Read the model definition and answer for the solid it produces. Units are mm, in the model's axes. A direction names the side the tool comes from. Give positions to 0.01 mm unless a question says otherwise; leave off trailing zeros. Order: outer loops, then holes, each group sorted by start corner. A loop starts at its lowest first (then second) coordinate and runs counter-clockwise, first axis right, second up.
```python
from build123d import *

# Parameters (mm, degrees)
F1_DEPTH      = 4.5
F2_DEPTH      = 4
F3_T          = -2.5
F4_R          = 1.52
F5_DEPTH      = 1.04
F6_R          = 1.52
F7_DEPTH      = 1.04
F8_R          = 1.52
F9_DEPTH      = 1.04
F10_R         = 1.52
F11_DEPTH     = 1.04
F12_R         = 1.52
F13_DEPTH     = 1.04
F14_R         = 1.52
F15_DEPTH     = 1.04
F16_T1_DEPTH  = 25.1433659759
F16_T3_DEPTH  = 25.1433659759
F16_T5_DEPTH  = 25.1433659759
F16_T7_DEPTH  = 25.1433659759
F16_T9_DEPTH  = 25.1433659759
F16_T11_DEPTH = 25.1433659759


# Not quite as in the source:
# - a fillet or chamfer that OpenCascade refuses, or shapes differently, is made with other operations: its cross-section is extruded or revolved along the edge and cut away or added


with BuildPart() as f1:
    # F0 (on Top) → F1 (new body)
    with BuildSketch(Plane.XY):
        Polygon((-8.9919036831, 15.2349256124), (-17.6897844467, -0.1697542118), (-8.6978807636, -15.4046798242), (8.9919036831, -15.2349256124), (17.6897844467, 0.1697542118), (8.6978807636, 15.4046798242), align=None)
    extrude(amount=F1_DEPTH)

    # F0 (on Top) → F2 (join)
    with BuildSketch(Plane.XY):
        Polygon((-19.9990791985, -0.1919146011), (-9.8333366793, -17.4156679387), (10.1657425191, -17.2237533376), (19.9990791985, 0.1919146011), (9.8333366793, 17.4156679387), (-10.1657425191, 17.2237533376), align=None)
        Polygon((-8.6978807636, -15.4046798242), (-17.6897844467, -0.1697542118), (-8.9919036831, 15.2349256124), (8.6978807636, 15.4046798242), (17.6897844467, 0.1697542118), (8.9919036831, -15.2349256124), align=None, mode=Mode.SUBTRACT)
    extrude(amount=F2_DEPTH)

    # F3
    f3_openings = [f1.faces().sort_by_distance(p)[0] for p in [
        (0, 0, 0),
    ]]
    offset(amount=F3_T, openings=f3_openings, kind=Kind.INTERSECTION)

    # F4 (on face) → F5 (cut)
    with BuildSketch(Plane(origin=(15.0824108588, -8.5159193683, 0), x_dir=(0.491666834, 0.8707833969, 0), z_dir=(0.8707833969, -0.491666834, 0))):
        with Locations((-6, 2)):
            Circle(F4_R)
        with Locations((6, 2)):
            Circle(F4_R)
    extrude(amount=-F5_DEPTH, mode=Mode.SUBTRACT)

    # F6 (on face) → F7 (cut)
    with BuildSketch(Plane(origin=(0.1662029199, -17.3197106382, 0), x_dir=(0.9999539599, 0.0095957301, 0), z_dir=(0.0095957301, -0.9999539599, 0))):
        with Locations((-6, 2)):
            Circle(F6_R)
        with Locations((6, 2)):
            Circle(F6_R)
    extrude(amount=-F7_DEPTH, mode=Mode.SUBTRACT)

    # F8 (on face) → F9 (cut)
    with BuildSketch(Plane(origin=(-14.9162079389, -8.8037912699, 0), x_dir=(0.508287126, -0.8611876669, 0), z_dir=(-0.8611876669, -0.508287126, 0))):
        with Locations((-6, 2)):
            Circle(F8_R)
        with Locations((6, 2)):
            Circle(F8_R)
    extrude(amount=-F9_DEPTH, mode=Mode.SUBTRACT)

    # F10 (on face) → F11 (cut)
    with BuildSketch(Plane(origin=(-15.0824108588, 8.5159193683, 0), x_dir=(-0.491666834, -0.8707833969, 0), z_dir=(-0.8707833969, 0.491666834, 0))):
        with Locations((-6, 2)):
            Circle(F10_R)
        with Locations((6, 2)):
            Circle(F10_R)
    extrude(amount=-F11_DEPTH, mode=Mode.SUBTRACT)

    # F12 (on face) → F13 (cut)
    with BuildSketch(Plane(origin=(-0.1662029199, 17.3197106382, 0), x_dir=(-0.9999539599, -0.0095957301, 0), z_dir=(-0.0095957301, 0.9999539599, 0))):
        with Locations((-6, 2)):
            Circle(F12_R)
        with Locations((6, 2)):
            Circle(F12_R)
    extrude(amount=-F13_DEPTH, mode=Mode.SUBTRACT)

    # F14 (on face) → F15 (cut)
    with BuildSketch(Plane(origin=(14.9162079389, 8.8037912699, 0), x_dir=(-0.508287126, 0.8611876669, 0), z_dir=(0.8611876669, 0.508287126, 0))):
        with Locations((-6, 2)):
            Circle(F14_R)
        with Locations((6, 2)):
            Circle(F14_R)
    extrude(amount=-F15_DEPTH, mode=Mode.SUBTRACT)

    # F16: chamfer of 1 on 6 edges, made by hand

    # F16_s2 → F16_t1 (cut)
    with BuildSketch(Plane(origin=(6.3900246144, -10.8265783412, 0), x_dir=(0, 0, 1), z_dir=(-0.508287126, 0.8611876669, 0))):
        Polygon((4, 16.3205080757), (3, 17.3205080757), (4, 17.3205080757), align=None)
    extrude(amount=F16_T1_DEPTH, mode=Mode.SUBTRACT)

    # F16_s4 → F16_t3 (cut)
    with BuildSketch(Plane(origin=(-6.1810795723, -10.9472128174, 0), x_dir=(0, 0, 1), z_dir=(0.491666834, 0.8707833969, 0))):
        Polygon((4, 16.3205080757), (3, 17.3205080757), (4, 17.3205080757), align=None)
    extrude(amount=F16_T3_DEPTH, mode=Mode.SUBTRACT)

    # F16_s6 → F16_t5 (cut)
    with BuildSketch(Plane(origin=(-12.5711041867, -0.1206344763, 0), x_dir=(0, 0, 1), z_dir=(0.9999539599, 0.0095957301, 0))):
        Polygon((4, 16.3205080757), (3, 17.3205080757), (4, 17.3205080757), align=None)
    extrude(amount=F16_T5_DEPTH, mode=Mode.SUBTRACT)

    # F16_s8 → F16_t7 (cut)
    with BuildSketch(Plane(origin=(-6.3900246144, 10.8265783412, 0), x_dir=(0, 0, 1), z_dir=(0.508287126, -0.8611876669, 0))):
        Polygon((4, 16.3205080757), (3, 17.3205080757), (4, 17.3205080757), align=None)
    extrude(amount=F16_T7_DEPTH, mode=Mode.SUBTRACT)

    # F16_s10 → F16_t9 (cut)
    with BuildSketch(Plane(origin=(6.1810795723, 10.9472128174, 0), x_dir=(0, 0, 1), z_dir=(-0.491666834, -0.8707833969, 0))):
        Polygon((4, 16.3205080757), (3, 17.3205080757), (4, 17.3205080757), align=None)
    extrude(amount=F16_T9_DEPTH, mode=Mode.SUBTRACT)

    # F16_s12 → F16_t11 (cut)
    with BuildSketch(Plane(origin=(12.5711041867, 0.1206344763, 0), x_dir=(0, 0, 1), z_dir=(-0.9999539599, -0.0095957301, 0))):
        Polygon((4, 16.3205080757), (3, 17.3205080757), (4, 17.3205080757), align=None)
    extrude(amount=F16_T11_DEPTH, mode=Mode.SUBTRACT)


solid = f1.part
```
1) Given pin 1 (13 mm diameter, centred on x = 0, y = 0.5, fed in from -Z); pin 2 (1.5 mm diameter, centred on x = -2, z = 3.5, fed in from -Y); pin 3 (1.5 mm diameter, centred on y = 3.5, z = 3.5, fed in from +X), each flat-ended and moving along its own axis, determine where each tip first touches the part or whether it passes through.
Final values:
pin 1: stops at z = 2
pin 2: stops at y = -17.35
pin 3: stops at x = 18.15
2) The part is cut by section A-A on y = -8.5. Determine the outline of the cut face in (x, z).
Final values:
outline: (-15.1, 0) - (-12.19, 0) - (-12.19, 1.5) - (-9.87, 1.5) - (-9.87, 2) - (9.92, 2) - (9.92, 1.5) - (12.22, 1.5) - (12.22, 0) - (15.09, 0) - (15.09, 3) - (13.94, 4) - (12.79, 4) - (12.79, 4.5) - (-12.77, 4.5) - (-12.77, 4) - (-13.93, 4) - (-15.1, 3) - close
3) For a pull along X with two mould halves and no side action, classify faces 1 (the face through (-14.57, 8.39, 3.51)), 2 (the face through (14.99, 8.68, 1.48)), 3 (the face through (-5.832, 16.753, 0.516)), 4 (the face through (-11.524, 13.775, 0.516)) as released by +X, released by -X, zero draft, split by the parting line, or undercut.
Final values:
face 1: released by -X
face 2: released by +X
face 3: undercut
face 4: undercut
4) Consider L1, parallel to Y at x = 7.5, z = 2.2; L2, parallel to Z at x = -7, y = 10.5; L3, parallel to Y at x = -7, z = 2.1. Determine where each line is inside the solid, lowest interval first.
Final values:
L1: y = -16.21 to 17.39
L2: z = 2 to 4.5
L3: y = -16.35 to 16.21
5) A tool of negligible diameter and unlimited length cuts with its end or side. For faces 5 (the face through (15.014, -8.638, 1.479)), 6 (the face through (13.257, 7.681, 4.246)), 7 (the face through (17.692, 3.092, 0.516)), 8 (the face through (12.847, -7.391, 0.74)), from which of +Z, -Z, +X, -X, +Y, -Y can it reach the whole face along a straight path? Write none if from no direction.
Final values:
face 5: +Z, -Z, +X, -Y
face 6: +Z, +X, +Y
face 7: none
face 8: -Z
